```python
from build123d import *

# Parameters (mm, degrees)
SKETCH1_R           = 15
BOSS_EXTRUDE1_DEPTH = 7.5
SKETCH2_R           = 1.5
BOSS_EXTRUDE2_DEPTH = 11
SKETCH4_R           = 7.5
CUT_EXTRUDE3_DEPTH  = 3.5
SKETCH6_R           = 1.5
CUT_EXTRUDE4_DEPTH  = 24.895606291


with BuildPart() as part:
    # Sketch1 → Boss-Extrude1 (new body)
    with BuildSketch(Plane(origin=(0, 0, 0), x_dir=(1, 0, 0), z_dir=(0, 1, 0))):
        with Locations(Location((0, 0, 0), (0, 0, 270))):
            Circle(SKETCH1_R)
    extrude(amount=BOSS_EXTRUDE1_DEPTH)

    # Sketch2 → Boss-Extrude2 (add)
    with BuildSketch(Plane(origin=(0, 7.5, 0), x_dir=(1, 0, 0), z_dir=(0, 1, 0))):
        with Locations(Location((0, 0, 0), (0, 0, 270))):
            Circle(SKETCH2_R)
    extrude(amount=BOSS_EXTRUDE2_DEPTH)

    # Sketch4 → Cut-Extrude3 (cut)
    with BuildSketch(Plane.XZ):
        with Locations(Location((0, 0, 0), (0, 0, 270))):
            Circle(SKETCH4_R)
    extrude(amount=-CUT_EXTRUDE3_DEPTH, mode=Mode.SUBTRACT)

    # Sketch6 → Cut-Extrude4 (cut, through all)
    with BuildSketch(Plane(origin=(0, 7.5, 0), x_dir=(1, 0, 0), z_dir=(0, 1, 0))):
        with Locations(Location((0, 11.5, 0), (0, 0, 270))):
            Circle(SKETCH6_R)
        with Locations(Location((11.5, 0, 0), (0, 0, 270))):
            Circle(SKETCH6_R)
        with Locations(Location((0, -11.5, 0), (0, 0, 270))):
            Circle(SKETCH6_R)
        with Locations(Location((-11.5, 0, 0), (0, 0, 270))):
            Circle(SKETCH6_R)
    extrude(amount=-CUT_EXTRUDE4_DEPTH, mode=Mode.SUBTRACT)


solid = part.part
```
Can you work these out from the model? Positions are in its coordinate system, mm. A direction names the side the tool comes from. Give positions to 0.01 mm unless a question says otherwise; leave off trailing zeros. Write each loop counter-clockwise with the first axis right and the second up, starting at its lowest first coordinate (ties: lowest second). Pieces come first, ordered by that corner, then holes. Notation, with made-up numbers: (-0.75, -20) -> (39.25, -20) arc R24 cw to (39.25, 0) -> close; hole circle Ø10 at (88, 0). An arc over 180 degrees is marked (long way). One line per item, written item: value.
Q1. Imagine slicing it at D-D on z = -12. Please give me the cut outline in (x, y).
Results found:
outline: (-9, 0) -> (-1.41, 0) -> (-1.41, 7.5) -> (-9, 7.5) -> close; (1.41, 0) -> (9, 0) -> (9, 7.5) -> (1.41, 7.5) -> close
Q2. Which directions (+Z, -Z, +X, -X, +Y, -Y) give clear straight access to the entire face, cutting with the end or side of a thin tool? Please do faces 4 (the face through (0.66, 3.698, -14.985)), 5 (the face through (0.33, 1.726, 7.493)).
Results found:
face 4: +Y, -Y
face 5: -Y
Q3. Imagine slicing it at C-C on z = 0. Please give me the cut outline in (x, y), and give its area (4 significant figures).
Results found:
outline: (-15, 0) -> (-13, 0) -> (-13, 7.5) -> (-15, 7.5) -> close; (-10, 0) -> (-7.5, 0) -> (-7.5, 3.5) -> (7.5, 3.5) -> (7.5, 0) -> (10, 0) -> (10, 7.5) -> (1.5, 7.5) -> (1.5, 18.5) -> (-1.5, 18.5) -> (-1.5, 7.5) -> (-10, 7.5) -> close; (13, 0) -> (15, 0) -> (15, 7.5) -> (13, 7.5) -> close
area: 160.5 mm^2
Q4. Please list where these lines run through material, in increasing order: line 1 (X direction, y = 5.25, z = 0); line 2 (Y direction, x = 8.75, z = 2.25); line 3 (X direction, y = 1.75, z = -4.5). Write a range as [from, to].
Results found:
line 1: x = [-15, -13], [-10, 10], [13, 15]
line 2: y = [0, 7.5]
line 3: x = [-14.31, -6], [6, 14.31]
Q5. We'd pull the mould along X, two halves only. Please class faces 1 (the face through (11.95, 3.8, 1.43)), 2 (the face through (0.45, 12.92, 1.43)), 3 (the face through (7, 0, -4)): +X half, -X half, draft (parallel to the pull), parting line (faces both ways), or undercut.
Results found:
face 1: undercut
face 2: parting line
face 3: draft
Q6. Imagine slicing it at B-B on y = 6.25. Please give me the cut outline in (x, z), and give its area (3 significant figures).
Results found:
outline: circle Ø30 at (0, 0); hole circle Ø3 at (-11.5, 0); hole circle Ø3 at (0, -11.5); hole circle Ø3 at (0, 11.5); hole circle Ø3 at (11.5, 0)
area: 679 mm^2
Q7. Imagine slicing it at A-A on x = 0. Please give me the cut outline in (y, z), and give its area (4 significant figures).
Results found:
outline: (0, -15) -> (7.5, -15) -> (7.5, -13) -> (0, -13) -> close; (0, -10) -> (7.5, -10) -> (7.5, -1.5) -> (18.5, -1.5) -> (18.5, 1.5) -> (7.5, 1.5) -> (7.5, 10) -> (0, 10) -> (0, 7.5) -> (3.5, 7.5) -> (3.5, -7.5) -> (0, -7.5) -> close; (0, 13) -> (7.5, 13) -> (7.5, 15) -> (0, 15) -> close
area: 160.5 mm^2
Q8. For P1, Ø1.8, axis at x = 11.5, z = 0, coming from the -Y side; P2, Ø2, axis at x = 4.5, z = -2.5, coming from the -Y side; P3, Ø4, axis at x = 11, y = 8, coming from the -Z side; P4, Ø4, axis at y = 2, z = -8.5, coming from the -X side, each with a flat end and sliding along its axis, tell me the tip position at first contact or that it passes through.
Results found:
P1: passes through
P2: stops at y = 3.5
P3: stops at z = -11.95
P4: stops at x = -13.52
